Autodesk Inventor part; units mm, degrees
ref_plane "YZ Plane" through (0, 0, 0) normal (1, 0, 0) x (0, 1, 0)
ref_plane "XZ Plane" through (0, 0, 0) normal (0, 1, 0) x (-1, 0, 0)
ref_plane "XY Plane" through (0, 0, 0) normal (0, 0, 1) x (1, 0, 0)
sketch "Sketch1" plane through (0, 0, 0) normal (0, 0, 1) x (1, 0, 0)
  point P0 (0, 0)
sketch "Sketch2" plane through (0, 0, 0) normal (0, 0, 1) x (1, 0, 0)
  line L0 (0.3174, 0) -> (65.5954, 0)
  line L1 (73.2154, 7.62) -> (73.2154, 31.242)
  line L2 (65.5954, 38.862) -> (0.3174, 38.862)
  line L3 (-7.3026, 31.242) -> (-7.3026, 7.62)
  arc A0 (0.3174, 38.862) -> (-7.3026, 31.242) centre (0.3174, 31.242) ccw
  arc A1 (-7.3026, 7.62) -> (0.3174, 0) centre (0.3174, 7.62) ccw
  arc A2 (73.2154, 31.242) -> (65.5954, 38.862) centre (65.5954, 31.242) ccw
  arc A3 (65.5954, 0) -> (73.2154, 7.62) centre (65.5954, 7.62) ccw
  point P0 (0, 0)
  point P1 (-7.3026, 0)
  point P2 (73.2154, 0)
  point P3 (73.2154, 38.862)
  dimension "d0" = 80.518
  dimension "d1" = 38.862
  dimension "d2" = 7.62
extrude "Extrusion1" add sketch "Sketch2" along normal blind 80.518
sketch "Sketch3" plane through (0, 0, 80.518) normal (0, 0, 1) x (1, 0, 0)
  line L0 (7.5564, 7.62) -> (58.3564, 7.62)
  line L1 (63.4364, 12.7) -> (63.4364, 26.162)
  line L2 (58.3564, 31.242) -> (7.5564, 31.242)
  line L3 (2.4764, 26.162) -> (2.4764, 12.7)
  line L4 (73.2154, 7.62) -> (73.2154, 31.242)
  line L5 (65.5954, 38.862) -> (0.3174, 38.862)
  arc A0 (7.5564, 31.242) -> (2.4764, 26.162) centre (7.5564, 26.162) ccw
  arc A1 (2.4764, 12.7) -> (7.5564, 7.62) centre (7.5564, 12.7) ccw
  arc A2 (58.3564, 7.62) -> (63.4364, 12.7) centre (58.3564, 12.7) ccw
  arc A3 (63.4364, 26.162) -> (58.3564, 31.242) centre (58.3564, 26.162) ccw
  point P0 (0, 0)
  point P1 (2.4764, 7.62)
  point P2 (63.4364, 7.62)
  point P3 (63.4364, 31.242)
  dimension "d5" = 60.96
  dimension "d6" = 23.622
  dimension "d7" = 9.779
  dimension "d8" = 7.62
  dimension "d9" = 5.08
extrude "Extrusion2" cut sketch "Sketch3" against normal blind 14.478
sketch "Sketch4" plane through (0.3174, 38.862, 0) normal (0, 1, 0) x (1, 0, 0)
  line L0 (12.573, -19.304) -> (52.705, -19.304)
  line L1 (57.785, -24.384) -> (57.785, -54.61)
  line L2 (52.705, -59.69) -> (12.573, -59.69)
  line L3 (7.493, -54.61) -> (7.493, -24.384)
  line L4 (65.278, -80.518) -> (0, -80.518)
  line L5 (72.898, 0) -> (72.898, -80.518)
  arc A0 (7.493, -54.61) -> (12.573, -59.69) centre (12.573, -54.61) ccw
  arc A1 (12.573, -19.304) -> (7.493, -24.384) centre (12.573, -24.384) ccw
  arc A2 (57.785, -24.384) -> (52.705, -19.304) centre (52.705, -24.384) ccw
  arc A3 (52.705, -59.69) -> (57.785, -54.61) centre (52.705, -54.61) ccw
  point P0 (-0.3174, 0)
  point P1 (7.493, -19.304)
  point P2 (57.785, -19.304)
  point P3 (57.785, -59.69)
  point P4 (7.493, -59.69)
  dimension "d12" = 50.292
  dimension "d13" = 40.386
  dimension "d14" = 20.828
  dimension "d15" = 15.113
  dimension "d18" = 5.08
extrude "Extrusion3" cut sketch "Sketch4" against normal blind 27.178
sketch "Sketch5" plane through (0, 0, 80.518) normal (0, 0, 1) x (1, 0, 0)
  line L0 (73.2154, 7.62) -> (73.2154, 31.242)
  line L1 (73.2154, 31.242) -> (71.6914, 31.242)
  line L2 (71.6914, 31.242) -> (71.6914, 29.718)
  line L3 (71.6914, 29.718) -> (73.2154, 29.718)
  line L4 (73.2154, 31.242) -> (73.2154, 29.718)
  line L5 (65.5954, 38.862) -> (0.3174, 38.862)
  point P0 (0, 0)
  dimension "d19" = 1.524
  dimension "d20" = 1.524
  dimension "d21" = 7.62
extrude "Extrusion4" cut sketch "Sketch5" against normal blind 80.518
sketch "Sketch6" plane through (0, 0, 80.518) normal (0, 0, 1) x (1, 0, 0)
  line L0 (-7.3026, 31.242) -> (-7.3026, 7.62)
  line L1 (-7.3026, 31.242) -> (-5.7786, 31.242)
  line L2 (-5.7786, 31.242) -> (-5.7786, 29.718)
  line L3 (-5.7786, 29.718) -> (-7.3026, 29.718)
  line L4 (-7.3026, 31.242) -> (-7.3026, 29.718)
  point P0 (0, 0)
  dimension "d24" = 1.524
  dimension "d25" = 1.524
extrude "Extrusion5" cut sketch "Sketch6" against normal blind 80.518
properties material "Wood (Cherry)"
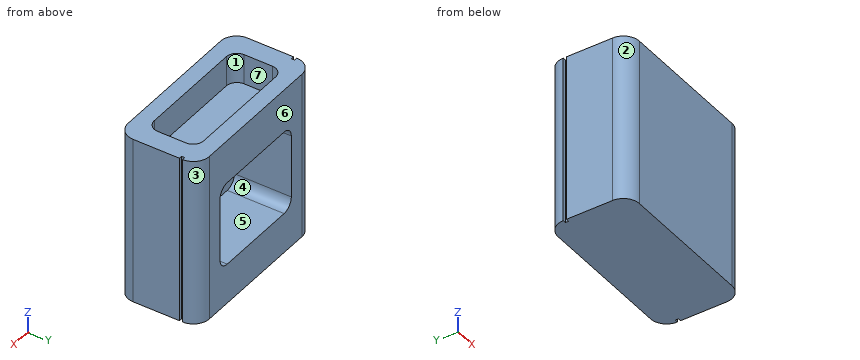
Can you work these out from the model? Positions are in its coordinate system, mm. Face numbers are marked on the shaded views. A direction names the side the tool comes from. Coordinates: 2 decimals unless noted, no trailing zeros. Order: outer loops, then holes, each group sorted by start corner. A loop starts at its lowest first (then second) coordinate and runs counter-clockwise, first axis right, second up. Notation, with made-up numbers: (68.25, 52) - (102.25, 52) arc R15 cw to (102.25, 79) - close; hole circle Ø5 at (51, 3). An arc over 180 degrees is marked (long way). Answer as a JSON object with one key per item and string values. Group by question number.
Q1. Imagine slicing it at B-B (y = 19.5). Please give me the cut outline in (x, z).
Q2. I need wall thicknesses on line 1 (Z direction, x = 34.5, y = 27); line 2 (X direction, y = 26, z = 53.5); line 3 (Y direction, x = 26, z = 75.5). Which ranges of each line are inside material? Lowest first, please. Write a range as from..to.
Q3. We'd pull the mould along Y, two halves only. Please class the marked faces 1, 2, 3 and 4: +Y half, -Y half, draft (parallel to the pull), parting line (faces both ways), or undercut.
Q4. Imagine slicing it at A-A (z = 74.5). Please give me the cut outline in (x, y).
Q5. Imagine slicing it at C-C (x = 32.5). Please give me the cut outline in (y, z), and give its area (3 significant figures).
Q6. Imagine slicing it at D-D (z = 61). Please give me the cut outline in (x, y), and give its area (3 significant figures).
Q7. On a 3-axis mill with a long thin cutter (end or side, diameter ignored), from which of +Z, -Z, +X, -X, +Y, -Y can I reach the whole of each face in a straight line? I mean the marked faces 5, 6 and 7. Say none if no direction works.
Q8. Will these pins go through, and if not, where does the flat tip stop? P1, Ø1.2, axis at x = 72, z = 52, coming from the +Y side; P2, Ø5, axis at x = 20.5, y = 12.5, coming from the +Z side; P3, Ø3, axis at x = 54.5, z = 52, coming from the +Y side.
Determined:
{
 "1": {"outline": "(-7.3, 0) - (73.22, 0) - (73.22, 80.52) - (63.44, 80.52) - (63.44, 66.04) - (2.48, 66.04) - (2.48, 80.52) - (-7.3, 80.52) - close; hole (7.81, 24.38) arc R5.08 ccw to (12.89, 19.3) - (53.02, 19.3) arc R5.08 ccw to (58.1, 24.38) - (58.1, 54.61) arc R5.08 ccw to (53.02, 59.69) - (12.89, 59.69) arc R5.08 ccw to (7.81, 54.61) - close"},
 "2": {"line 1": "z = 0..19.3, 59.69..66.04", "line 2": "x = -7.3..7.81, 58.1..73.22", "line 3": "y = 0..7.62, 31.24..38.86"},
 "3": {"face 1": "undercut", "face 2": "-Y half", "face 3": "+Y half", "face 4": "draft"},
 "4": {"outline": "(-7.3, 7.62) arc R7.62 ccw to (0.32, 0) - (65.6, 0) arc R7.62 ccw to (73.22, 7.62) - (73.22, 29.72) - (71.69, 29.72) - (71.69, 31.24) - (73.22, 31.24) arc R7.62 ccw to (65.6, 38.86) - (0.32, 38.86) arc R7.62 ccw to (-7.3, 31.24) - (-5.78, 31.24) - (-5.78, 29.72) - (-7.3, 29.72) - close; hole (2.48, 12.7) arc R5.08 ccw to (7.56, 7.62) - (58.36, 7.62) arc R5.08 ccw to (63.44, 12.7) - (63.44, 26.16) arc R5.08 ccw to (58.36, 31.24) - (7.56, 31.24) arc R5.08 ccw to (2.48, 26.16) - close"},
 "5": {"outline": "(0, 0) - (38.86, 0) - (38.86, 19.3) - (11.68, 19.3) - (11.68, 59.69) - (38.86, 59.69) - (38.86, 80.52) - (31.24, 80.52) - (31.24, 66.04) - (7.62, 66.04) - (7.62, 80.52) - (0, 80.52) - close", "area": "1,690 mm2"},
 "6": {"outline": "(-7.3, 7.62) arc R7.62 ccw to (0.32, 0) - (65.6, 0) arc R7.62 ccw to (73.22, 7.62) - (73.22, 29.72) - (71.69, 29.72) - (71.69, 31.24) - (73.22, 31.24) arc R7.62 ccw to (65.6, 38.86) - (0.32, 38.86) arc R7.62 ccw to (-7.3, 31.24) - (-5.78, 31.24) - (-5.78, 29.72) - (-7.3, 29.72) - close", "area": "3,070 mm2"},
 "7": {"face 5": "+Y", "face 6": "+Z, -Z, +X, -X, +Y", "face 7": "+Z"},
 "8": {"P1": "stops at y = 36.18", "P2": "stops at z = 66.04", "P3": "stops at y = 11.68"}
}
